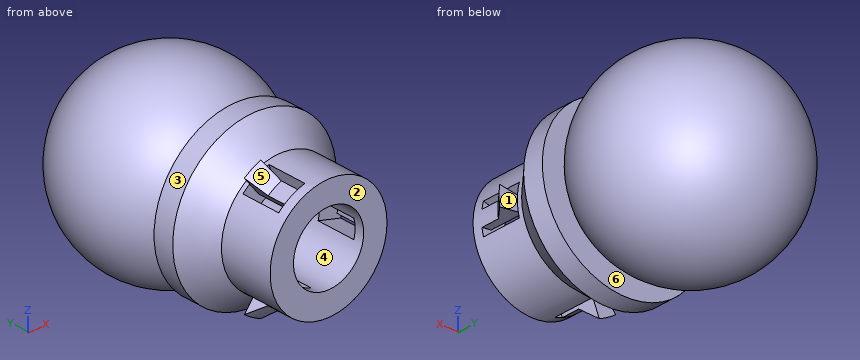
from build123d import *
from build123d import SkipClean  # not in build123d's __all__

# Parameters (mm, degrees)
F0_W            = 5
F0_H            = 4.387505004
F3_ANGLE_BACK   = 15
F3_ANGLE        = 30
F3_COPIES_COUNT = 3
F4_ANGLE_BACK   = 7.5
F4_ANGLE        = 15
F4_COPIES_COUNT = 3


# Not quite as in the source:
# - a pattern or mirror of a feature is missing from the dataset's text; its kind, count and spacing are read off the source's solid


with BuildPart() as f1:
    # F0 (on Top) → F1 (revolve)
    with BuildSketch(Plane.XY):
        with BuildLine():
            ThreePointArc((12.5, 21.7588313682), (18.8712731409, 43.9951507913), (0, 57.3713263642))
            Line((0, 57.3713263642), (0, 52.3713263642))
            ThreePointArc((0, 52.3713263642), (14.4888873943, 41.2536120408), (7.5, 24.3809453075))
            Line((7.5, 24.3809453075), (7.5, 18.8308301465))
            ThreePointArc((7.5, 18.8308301465), (10.1065967461, 20.1128008707), (12.5, 21.7588313682))
        make_face()
        with BuildLine():
            Line((12.5, 17.3713263642), (12.5, 21.7588313682))
            ThreePointArc((12.5, 21.7588313682), (10.1065967461, 20.1128008707), (7.5, 18.8308301465))
            Line((7.5, 18.8308301465), (7.5, 0))
            Line((7.5, 0), (12.5, 0))
            Line((12.5, 0), (12.5, 11.4125584013))
            Line((12.5, 11.4125584013), (12.5, 17.3713263642))
        make_face()
        with Locations((15, 19.5650788662)):
            Rectangle(F0_W, F0_H)
        Polygon((17.5, 17.3713263642), (12.5, 17.3713263642), (12.5, 11.4125584013), align=None)
    revolve(axis=Axis((0, 26.1856631821, 0), (0, 1, 0)))

    # F2 (on Top) → F3 (revolve, cut)
    with BuildSketch(Plane.XY, mode=Mode.PRIVATE) as f3_sk:
        Polygon((7.5, 10.4125584013), (7.5, 2), (10.5, 2), (10.5, 9.4125584013), (12.5, 9.4125584013), (12.5, 10.4125584013), align=None)
        Polygon((10.5, 2), (12.5, 2), (12.5, 5.8372976235), (12.5, 9.4125584013), (10.5, 9.4125584013), align=None)
    f3 = revolve(f3_sk.sketch.rotate(Axis((0, 0, 0), (0, -1, 0)), -F3_ANGLE_BACK), axis=Axis((0, 0, 0), (0, -1, 0)), revolution_arc=F3_ANGLE, mode=Mode.SUBTRACT)

    # F3_copies: F3 ×3 about axis
    f3_copies_axis = Axis((0, 0, 0), (0, 1, 0))
    for i in range(1, F3_COPIES_COUNT):
        add(f3.rotate(f3_copies_axis, i * 360 / F3_COPIES_COUNT), clean=False, mode=Mode.SUBTRACT)

    # F2 (on Top) → F4 (revolve)
    with BuildSketch(Plane.XY, mode=Mode.PRIVATE) as f4_sk:
        Polygon((12.5, 9.4125584013), (12.5, 5.8372976235), (15.5, 9.4125584013), align=None)
        Polygon((10.5, 2), (12.5, 2), (12.5, 5.8372976235), (12.5, 9.4125584013), (10.5, 9.4125584013), align=None)
    f4 = revolve(f4_sk.sketch.rotate(Axis((0, 0, 0), (0, 1, 0)), -F4_ANGLE_BACK), axis=Axis((0, 0, 0), (0, 1, 0)), revolution_arc=F4_ANGLE)

    # F4_copies: F4 ×3 about axis
    f4_copies_axis = Axis((0, 0, 0), (0, 1, 0))
    with SkipClean():  # cleaning this boolean's faces spoils the solid; the shape is the same uncleaned
        for i in range(1, F4_COPIES_COUNT):
            add(f4.rotate(f4_copies_axis, i * 360 / F4_COPIES_COUNT), clean=False)


solid = f1.part
CAD build for the part. Positions are in the model's coordinates, mm. Face numbers are marked on the shaded views. A direction names the side the tool comes from. Give positions to 0.01 mm unless a question says otherwise; leave off trailing zeros. Loops run counter-clockwise (first coordinate to the right, second up) from the corner with the lowest first, then second, coordinate; pieces in that order, holes last. Notation, with made-up numbers: M -37,0.25 L -16,0.25 A17 cw -16,30.25 Z; hole C 0.25,48 d5. An arc over 180 degrees is marked long. Answer in a Markdown table with one row per item. Add a question column.
Item 1: Band-saw the part on C-C on y = 48. Give the cut face in (x, z), then the cut area to 3 significant figures.
Item 2: Drop flat-ended pins along their axis: P1, Ø5, axis at x = 12.5, z = 14, coming from the -Y side; P2, Ø12, axis at x = 2.5, y = 30, coming from the -Z side; P3, Ø1.5, axis at y = 10.5, z = -14, coming from the -X side; P4, Ø6, axis at x = 14.5, z = 9.5, coming from the +Y side. Give the stop position or say it passes through.
Item 3: Tool access for the marked faces 4, 5 and 6: list every direction of +Z, -Z, +X, -X, +Y, -Y with a clear straight run to the whole face (end or side of a thin tool).
Item 4: Mould opens along Y. For the marked faces 1, 2 and 3 say: +Y half, -Y half, draft (parallel to the pull), parting line (faces both ways), or undercut.
Item 5: Band-saw the part on A-A on z = 0. Give the cut face in (x, y).
Item 6: Band-saw the part on B-B on x = 0. Give the cut face in (y, z), then the cut area to 3 significant figures.
Item 7: Probe probe 1 along Z at (x, y) = (0, 11.25); probe 2 along Z at (x, y) = (-0.5, 22.5); probe 3 along X at (y, z) = (17.25, 0). List the from-to ranges inside material, lowest first.
Reply:
| question | item | result |
|---|---|---|
| 1 | outline | C 0,0 d33.88; hole C 0,0 d21.17 |
| 1 | area | 550 mm^2 |
| 2 | P1 | stops at y = 15.9 |
| 2 | P2 | stops at z = -19.92 |
| 2 | P3 | passes through |
| 2 | P4 | stops at y = 51.32 |
| 3 | face 4 | -Y |
| 3 | face 5 | +Z, -X, -Y |
| 3 | face 6 | none |
| 4 | face 1 | undercut |
| 4 | face 2 | -Y half |
| 4 | face 3 | draft |
| 5 | outline | M -17.5,17.37 L -12.5,11.41 L -12.5,0 L -7.5,0 L -7.5,24.38 A15 cw long 7.5,24.38 L 7.5,10.41 L 12.5,10.41 L 12.5,11.41 L 17.5,17.37 L 17.5,21.76 L 12.5,21.76 A20 ccw long -12.5,21.76 L -17.5,21.76 Z; M 7.5,0 L 12.5,0 L 12.5,5.84 L 15.5,9.41 L 10.5,9.41 L 10.5,2 L 7.5,2 Z |
| 6 | outline | M 0,-12.5 L 11.41,-12.5 L 17.37,-17.5 L 21.76,-17.5 L 21.76,-12.5 A20 ccw long 21.76,12.5 L 21.76,17.5 L 17.37,17.5 L 11.41,12.5 L 0,12.5 L 0,7.5 L 24.38,7.5 A15 cw long 24.38,-7.5 L 0,-7.5 Z |
| 6 | area | 747 mm^2 |
| 7 | probe 1 | z = -12.5 to -7.5, 7.5 to 12.5 |
| 7 | probe 2 | z = -13.36 to -7.48, 7.48 to 13.36 |
| 7 | probe 3 | x = -17.4 to -7.5, 7.5 to 17.4 |
